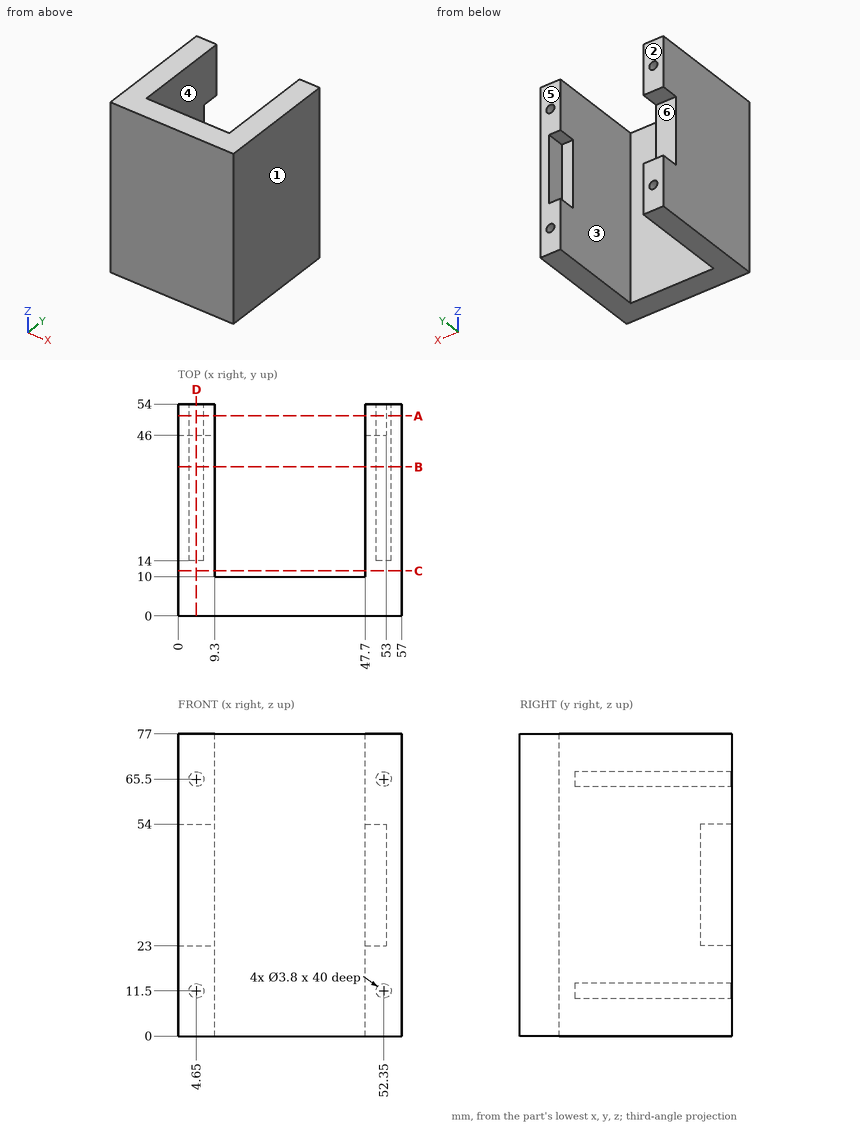
Can you work these out from the drawing? Everything is in mm from the part's minimum corner. A direction names the side the tool comes from. Coordinates: 2 decimals unless noted, no trailing zeros. Loops run counter-clockwise (first coordinate to the right, second up) from the corner with the lowest first, then second, coordinate; pieces in that order, holes last. Notation, with made-up numbers: M 25,10.25 L 81,10.25 A30 ccw 81,38.25 Z; hole C -18,-1 d2. An arc over 180 degrees is marked long. One line per item, written item: value.
1. Imagine slicing it at C-C (y = 11.5). List the corners of the cut face in (x, z) for me.
Geometry says:
outline: M 0,0 L 9.3,0 L 9.3,77 L 0,77 Z; M 47.7,0 L 57,0 L 57,77 L 47.7,77 Z
2. Imagine slicing it at B-B (y = 38). List the corners of the cut face in (x, z) for me.
Geometry says:
outline: M 0,0 L 9.3,0 L 9.3,77 L 0,77 Z; M 47.7,0 L 57,0 L 57,77 L 47.7,77 Z; hole C 4.65,11.5 d3.8; hole C 4.65,65.5 d3.8; hole C 52.35,11.5 d3.8; hole C 52.35,65.5 d3.8
3. Imagine slicing it at A-A (y = 51). List the corners of the cut face in (x, z) for me, and give its area (3 significant figures).
Geometry says:
outline: M 0,0 L 9.3,0 L 9.3,23 L 0,23 Z; M 0,54 L 9.3,54 L 9.3,77 L 0,77 Z; M 47.7,0 L 57,0 L 57,77 L 47.7,77 L 47.7,54 L 53,54 L 53,23 L 47.7,23 Z; hole C 4.65,11.5 d3.8; hole C 4.65,65.5 d3.8; hole C 52.35,11.5 d3.8; hole C 52.35,65.5 d3.8
area: 934 mm2
4. Will these pins go through, and if not, where does the flat tip stop? pin 1 Ø6 at (x, z) = (36.5, 33) entering from +Y; pin 2 Ø5 at (x, z) = (50, 41) entering from +Y; pin 3 Ø4.5 at (x, z) = (52.35, 11.5) entering from -Y; pin 4 Ø1.9 at (x, z) = (4, 12) entering from +Y.
Geometry says:
pin 1: stops at y = 10
pin 2: stops at y = 46
pin 3: stops at y = 0
pin 4: stops at y = 14
5. On a 3-axis mill with a long thin cutter (end or side, diameter ignored), from which of +Z, -Z, +X, -X, +Y, -Y can I reach the whole of each face in a straight line? I mean the marked faces 4, 5 and 6. Say none if no direction works.
Geometry says:
face 4: +Z, -Z, +Y
face 5: +Z, -Z, +X, -X, +Y
face 6: -X, +Y
6. Please list where these lines run through material, in increasing order: probe 1 along X at (y, z) = (45, 65.5); probe 2 along X at (y, z) = (21, 18); probe 3 along Z at (x, y) = (52, 23).
Geometry says:
probe 1: x = 0 to 2.75, 6.55 to 9.3, 47.7 to 50.45, 54.25 to 57
probe 2: x = 0 to 9.3, 47.7 to 57
probe 3: z = 0 to 9.63, 13.37 to 63.63, 67.37 to 77
7. Thinking about a two-plate mould opening in X: for the marked faces 1, 2 and 3, which applies, +X half, -X half, draft (parallel to the pull), parting line (faces both ways), or undercut?
Geometry says:
face 1: +X half
face 2: draft
face 3: undercut
8. Imagine slicing it at D-D (x = 4.65). List the corners of the cut face in (y, z) for me, and give its area (3 significant figures).
Geometry says:
outline: M 0,0 L 54,0 L 54,9.6 L 14,9.6 L 14,13.4 L 54,13.4 L 54,23 L 46,23 L 46,54 L 54,54 L 54,63.6 L 14,63.6 L 14,67.4 L 54,67.4 L 54,77 L 0,77 Z
area: 3,610 mm2
